The model under review builds one solid part; all positions refer to its coordinate system, in mm. Face numbers are marked on the shaded views. Coordinates: 2 decimals unless noted, no trailing zeros. Write each loop counter-clockwise with the first axis right and the second up, starting at its lowest first coordinate (ties: lowest second). Pieces come first, ordered by that corner, then holes. Notation, with made-up numbers: M -19.75,18.25 L 1.25,18.25 A19 cw 1.25,37.25 Z; hole C -37,-15 d10. An arc over 180 degrees is marked long. Answer as a JSON object with one key per item and string values.
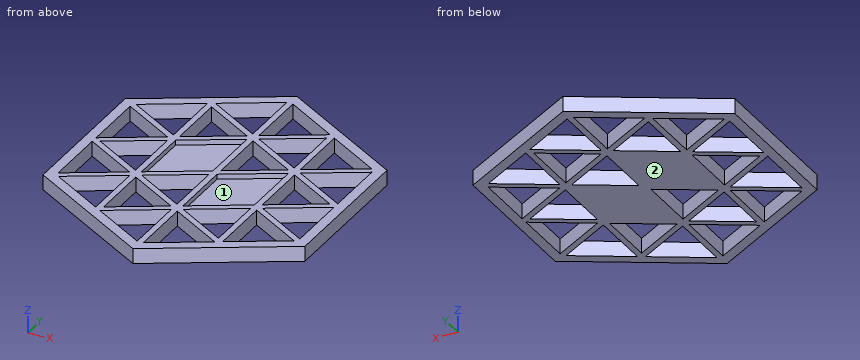
```python
from build123d import *

# Parameters (mm, degrees)
F1_DEPTH = 3
F3_DEPTH = 2


with BuildPart() as f1:
    # F0 (on Top) → F1 (new body)
    with BuildSketch(Plane.XY):
        Polygon((25.980762, 15), (0, 30), (-25.980762, 15), (-25.980762, -15), (0, -30), (25.980762, -15), align=None)
        Polygon((-0.6, -14.88453), (-0.6, -27.344189), (-11.390381, -21.114359), align=None, mode=Mode.SUBTRACT)
        Polygon((-12.590381, -7.96188), (-12.590381, -20.421539), (-23.380762, -14.19171), align=None, mode=Mode.SUBTRACT)
        Polygon((-13.190381, -6.92265), (-23.980762, -13.152479), (-23.980762, -0.69282), align=None, mode=Mode.SUBTRACT)
        Polygon((-12.590381, -5.883419), (-22.780762, 0), (-12.590381, 5.883419), align=None, mode=Mode.SUBTRACT)
        Polygon((-1.2, -13.845299), (-11.390381, -19.728719), (-11.390381, -7.96188), align=None, mode=Mode.SUBTRACT)
        Polygon((-0.6, -1.03923), (-0.6, -12.806069), (-10.790381, -6.92265), align=None, mode=Mode.SUBTRACT)
        Polygon((0.6, -14.88453), (11.390381, -21.114359), (0.6, -27.344189), align=None, mode=Mode.SUBTRACT)
        Polygon((11.390381, -7.96188), (11.390381, -19.728719), (1.2, -13.845299), align=None, mode=Mode.SUBTRACT)
        Polygon((0.6, -12.806069), (0.6, -0.34641), (11.390381, 5.883419), (11.390381, -6.57624), align=None, mode=Mode.SUBTRACT)
        Polygon((12.590381, -7.96188), (23.380762, -14.19171), (12.590381, -20.421539), align=None, mode=Mode.SUBTRACT)
        Polygon((13.190381, -6.92265), (23.980762, -0.69282), (23.980762, -13.152479), align=None, mode=Mode.SUBTRACT)
        Polygon((-13.190381, 6.92265), (-23.980762, 0.69282), (-23.980762, 13.152479), align=None, mode=Mode.SUBTRACT)
        Polygon((-12.590381, 7.96188), (-23.380762, 14.19171), (-12.590381, 20.421539), align=None, mode=Mode.SUBTRACT)
        Polygon((-0.6, 12.806069), (-0.6, 0.34641), (-11.390381, -5.883419), (-11.390381, 6.57624), align=None, mode=Mode.SUBTRACT)
        Polygon((-11.390381, 19.728719), (-1.2, 13.845299), (-11.390381, 7.96188), align=None, mode=Mode.SUBTRACT)
        Polygon((-0.6, 14.88453), (-11.390381, 21.114359), (-0.6, 27.344189), align=None, mode=Mode.SUBTRACT)
        Polygon((0.6, 12.806069), (10.790381, 6.92265), (0.6, 1.03923), align=None, mode=Mode.SUBTRACT)
        Polygon((11.390381, 19.728719), (11.390381, 7.96188), (1.2, 13.845299), align=None, mode=Mode.SUBTRACT)
        Polygon((12.590381, 5.883419), (22.780762, 0), (12.590381, -5.883419), align=None, mode=Mode.SUBTRACT)
        Polygon((13.190381, 6.92265), (23.980762, 13.152479), (23.980762, 0.69282), align=None, mode=Mode.SUBTRACT)
        Polygon((12.590381, 7.96188), (12.590381, 20.421539), (23.380762, 14.19171), align=None, mode=Mode.SUBTRACT)
        Polygon((0.6, 14.88453), (0.6, 27.344189), (11.390381, 21.114359), align=None, mode=Mode.SUBTRACT)
    extrude(amount=F1_DEPTH)

    # F2 (on face) → F3 (join)
    with BuildSketch(Plane(origin=(0, 0, 0), x_dir=(1, 0, 0), z_dir=(0, 0, -1))):
        Polygon((-11.390381, -6.57624), (-0.6, -12.806069), (-0.6, -0.34641), (-11.390381, 5.883419), align=None)
        Polygon((0.6, 0.34641), (11.390381, -5.883419), (11.390381, 6.57624), (0.6, 12.806069), align=None)
    extrude(amount=-F3_DEPTH)


solid = f1.part
```
(1) Add section B-B on x = 7. Give the boundary of the cut face in (y, z).
Results list:
{"outline": "M -25.96,0 L -23.65,0 L -23.65,3 L -25.96,3 Z; M -18.58,0 L -17.19,0 L -17.19,3 L -18.58,3 Z; M -10.5,0 L 4.73,0 L 4.73,3 L 3.35,3 L 3.35,2 L -9.11,2 L -9.11,3 L -10.5,3 Z; M 9.11,0 L 10.5,0 L 10.5,3 L 9.11,3 Z; M 17.19,0 L 18.58,0 L 18.58,3 L 17.19,3 Z; M 23.65,0 L 25.96,0 L 25.96,3 L 23.65,3 Z"}
(2) Add section A-A on y = -25. Give the boundary of the cut face in (x, z).
Results list:
{"outline": "M -8.66,0 L -4.66,0 L -4.66,3 L -8.66,3 Z; M -0.6,0 L 0.6,0 L 0.6,3 L -0.6,3 Z; M 4.66,0 L 8.66,0 L 8.66,3 L 4.66,3 Z"}
(3) Wall thickness on line 1 along X through (y, z) = (14, 2.75); line 2 along X through (y, z) = (-27, 1.25); line 3 along Y through (x, z) = (11, 1.7): over which ranges is each line inside the solid? List them lowest first. Write a range as from..to.
Results list:
{"line 1": "-25.98..-23.05, -12.59..-11.39, -1.47..1.47, 11.39..12.59, 23.05..25.98", "line 2": "-5.2..-1.2, -0.6..0.6, 1.2..5.2", "line 3": "-23.65..-21.34, -20.89..-19.5, -8.19..8.19, 19.5..20.89, 21.34..23.65"}
(4) For pin 1 Ø0.9 at (y, z) = (-19, 1) entering from +X; pin 2 Ø1.5 at (x, z) = (-10, 1.5) entering from -Y; pin 3 Ø1.5 at (x, z) = (10.5, 1.5) entering from -Y; pin 4 Ø2 at (x, y) = (15.5, -3) entering from -Z, all flat-tipped, find the tip position at first contact; note any pin that passes through.
Results list:
{"pin 1": "x = 19.83", "pin 2": "y = -24.66", "pin 3": "y = -24.37", "pin 4": "through"}
(5) Add section C-C on y = 4. Count the separate pieces of the cut face and the enclosed holes in it, and give its area (3 significant figures).
Results list:
{"separate pieces": "6", "enclosed holes": "0", "area": "72.5 mm²"}
(6) Draft analysis for pull direction X (two halves, no side actions). For the marked faces 1 and 2, state which applies: released by +X, released by -X, zero draft, split by the parting line, or undercut.
Results list:
{"face 1": "undercut", "face 2": "zero draft"}
